```python
from build123d import *

# Parameters (mm, degrees)
SKETCH4_W           = 7
SKETCH4_H           = 7
SKETCH4_R           = 1.25
BOSS_EXTRUDE2_DEPTH = 2.5


with BuildPart() as part:
    # Sketch4 → Boss-Extrude2 (new body)
    # profile 1 of 2: a face of its own
    with BuildSketch(Plane(origin=(0, 0, 0), x_dir=(1, 0, 0), z_dir=(0, 1, 0))):
        with Locations((-3.5, 3.5)):
            Rectangle(SKETCH4_W, SKETCH4_H)
        with Locations(Location((-3.5, 3, 0), (0, 0, 270))):
            Circle(SKETCH4_R, mode=Mode.SUBTRACT)
    # profile 2 of 2: a face of its own
    with BuildSketch(Plane(origin=(0, 0, 0), x_dir=(1, 0, 0), z_dir=(0, 1, 0))):
        Polygon((-7, 7), (0, 7), (8, 7), (8, 10), (-7, 10), align=None)
    extrude(amount=BOSS_EXTRUDE2_DEPTH)


solid = part.part
```
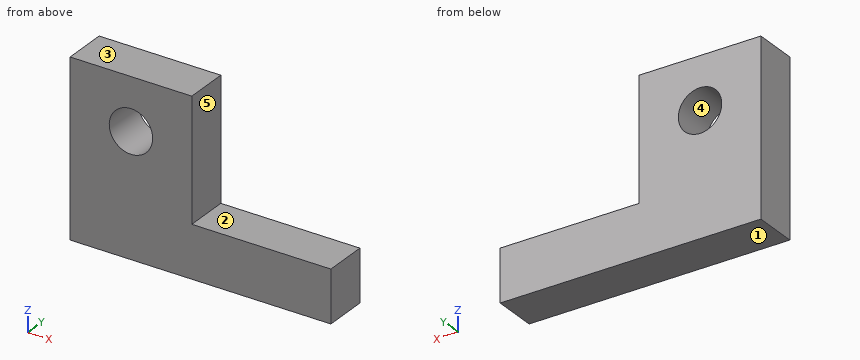
CAD build for the part. Positions are in the model's coordinates, mm. Face numbers are marked on the shaded views. A direction names the side the tool comes from. Coordinates: 2 decimals unless noted, no trailing zeros. Write each loop counter-clockwise with the first axis right and the second up, starting at its lowest first coordinate (ties: lowest second). Pieces come first, ordered by that corner, then holes. Notation, with made-up numbers: (49.25, -40) -> (81.25, -40) arc R31 cw to (81.25, -13) -> close; hole circle Ø4 at (20.25, 25.5). An arc over 180 degrees is marked (long way). Use CSV: the item, a comma, the result in double quotes. Start each with the question number.
Item 1: Band-saw the part on D-D, the plane z = -4.75. Write the cut outline in (x, y), plus the area to 3 significant figures.
Item 2: Band-saw the part on A-A, the plane x = -3.5. Write the cut outline in (y, z), plus the area to 4 significant figures.
Item 3: Two-plate mould, pull along X, no slides. Class the marked faces 3, 4 and 5: +X half, -X half, draft (parallel to the pull), parting line (faces both ways), or undercut.
Item 4: Tool access for the marked faces 1 and 2: list every direction of +Z, -Z, +X, -X, +Y, -Y with a clear straight run to the whole face (end or side of a thin tool).
Item 5: Band-saw the part on B-B, the plane z = -3. Write the cut outline in (x, y).
Item 6: Wall check: probe 1 along X at (y, z) = (0.7, -3); probe 2 along X at (y, z) = (0.4, -6.25); probe 3 along Z at (x, y) = (6, 1.1). Give the ranges that are in metal, low to high.
Item 7: Band-saw the part on C-C, the plane y = 0.3. Write the cut outline in (x, z).
Response values:
1,outline,"(-7, 0) -> (0, 0) -> (0, 2.5) -> (-7, 2.5) -> close"
1,area,"17.5 mm2"
2,outline,"(0, -10) -> (2.5, -10) -> (2.5, -4.25) -> (0, -4.25) -> close; (0, -1.75) -> (2.5, -1.75) -> (2.5, 0) -> (0, 0) -> close"
2,area,"18.75 mm2"
3,face 3,"draft"
3,face 4,"undercut"
3,face 5,"+X half"
4,face 1,"-Z, +X, -X, +Y, -Y"
4,face 2,"+Z, +X, +Y, -Y"
5,outline,"(-7, 0) -> (-4.75, 0) -> (-4.75, 2.5) -> (-7, 2.5) -> close; (-2.25, 0) -> (0, 0) -> (0, 2.5) -> (-2.25, 2.5) -> close"
6,probe 1,"x = -7 to -4.75, -2.25 to 0"
6,probe 2,"x = -7 to 0"
6,probe 3,"z = -10 to -7"
7,outline,"(-7, -10) -> (8, -10) -> (8, -7) -> (0, -7) -> (0, 0) -> (-7, 0) -> close; hole circle Ø2.5 at (-3.5, -3)"
